from build123d import *

# Parameters (mm, degrees)
F0_W      = 600
F0_H      = 540
F1_DEPTH  = 140
F2_W      = 200
F2_H      = 200
F3_DEPTH  = 140.001
F4_W      = 600
F4_H      = 240
F5_DEPTH  = 540
F6_W      = 300
F6_H      = 560
F7_DEPTH  = 140
F9_R      = 75
F10_DEPTH = 100.001
F8_R      = 150
F11_DEPTH = 140


with BuildPart() as f1:
    # F0 (on Top) → F1 (new body)
    with BuildSketch(Plane.XY):
        Rectangle(F0_W, F0_H)
    extrude(amount=F1_DEPTH)

    # F2 (on face) → F3 (cut, through all)
    with BuildSketch(Plane.XY.offset(140)):
        with Locations((0, -170)):
            Rectangle(F2_W, F2_H)
    extrude(amount=-F3_DEPTH, mode=Mode.SUBTRACT)

    # F4 (on face) → F5 (join)
    with BuildSketch(Plane.XY.offset(140)):
        with Locations((0, 150)):
            Rectangle(F4_W, F4_H)
    extrude(amount=F5_DEPTH)

    # F6 (on face) → F7 (cut)
    with BuildSketch(Plane.XZ.offset(-30)):
        with Locations((0, 680)):
            Rectangle(F6_W, F6_H)
    extrude(amount=-F7_DEPTH, mode=Mode.SUBTRACT)

    # F9 (on face) → F10 (cut, through all)
    with BuildSketch(Plane.XZ.offset(-170)):
        with Locations((0, 400)):
            Circle(F9_R)
    extrude(amount=-F10_DEPTH, mode=Mode.SUBTRACT)

    # F8 (on face) → F11 (cut)
    with BuildSketch(Plane.XZ.offset(-30)):
        with Locations((0, 400)):
            Circle(F8_R)
    extrude(amount=-F11_DEPTH, mode=Mode.SUBTRACT)


solid = f1.part
Check sheet for the modelled part. Datum: model origin and axes. Units: mm. A direction names the side the tool comes from. Coordinates: 2 decimals unless noted, no trailing zeros. Write each loop counter-clockwise with the first axis right and the second up, starting at its lowest first coordinate (ties: lowest second). Pieces come first, ordered by that corner, then holes. Notation, with made-up numbers: M 7,-19 L 35,-19 A36 ccw 35,15 Z; hole C 1.25,-2.5 d3. An arc over 180 degrees is marked long. Answer as CSV lines item,"result".
Q1. Cross-section at A-A (x = 0). Record the boundary of the cut face in (y, z).
Check result:
outline,"M -70,0 L 270,0 L 270,325 L 170,325 L 170,250 L 30,250 L 30,140 L -70,140 Z; M 170,475 L 270,475 L 270,680 L 170,680 Z"
Q2. Cross-section at B-B (y = -90). Record the boundary of the cut face in (x, z).
Check result:
outline,"M -300,0 L -100,0 L -100,140 L -300,140 Z; M 100,0 L 300,0 L 300,140 L 100,140 Z"
Q3. Cross-section at C-C (z = 541). Record the boundary of the cut face in (x, y), then the cut area to 3 significant figures.
Check result:
outline,"M -300,30 L -150,30 L -150,170 L 150,170 L 150,30 L 300,30 L 300,270 L -300,270 Z"
area,"102,000 mm^2"
Q4. Material ranges on probe 1 along X at (y, z) = (192.5, 400); probe 2 along Z at (x, y) = (0, 221); probe 3 along X at (y, z) = (-182, 43), recorded low to high. Write a range as from..to.
Check result:
probe 1,"-300..-75, 75..300"
probe 2,"0..325, 475..680"
probe 3,"-300..-100, 100..300"
Q5. Mould release check, pull along X, two halves, no side actions. Record for faces 1 (the face through (-300, 116, 260)), 2 (the face through (-4, 4, 0)), 3 (the face through (150, 99, 538)), 4 (the face through (-3.298, 99.02, 250.036)): released by +X, released by -X, zero draft, split by the parting line, or undercut.
Check result:
face 1,"released by -X"
face 2,"zero draft"
face 3,"undercut"
face 4,"undercut"
Q6. Go/stop test with flat-tipped pins: pin 1 (8 mm diameter, centred on x = 103.5, y = -40, fed in from +Z); pin 2 (8 mm diameter, centred on x = 156, z = 511.5, fed in from -Y); pin 3 (12 mm diameter, centred on x = -140.5, z = 529, fed in from -Y). Record where each tip stops, or that it passes through.
Check result:
pin 1,"z = 140"
pin 2,"y = 30"
pin 3,"y = 170"
Q7. Cross-section at D-D (y = 127). Record the boundary of the cut face in (x, z), then the cut area to 3 significant figures.
Check result:
outline,"M -300,0 L 300,0 L 300,680 L 150,680 L 150,400 A150 cw -150,400 L -150,680 L -300,680 Z"
area,"289,000 mm^2"
Q8. Set-up check for faces 5 (the face through (-100, -171, 71)), 6 (the face through (300, 116, 260)), 7 (the face through (-4, 30, 226)), 8 (the face through (-150, 99, 538)): record each of +Z, -Z, +X, -X, +Y, -Y from which the full face is reachable in a straight line by a thin tool's end or side.
Check result:
face 5,"+Z, -Z, -Y"
face 6,"+Z, -Z, +X, +Y, -Y"
face 7,"+Z, +X, -X, -Y"
face 8,"+Z, -Y"
